```python
from build123d import *

# Parameters (mm, degrees)
F0_W      = 132.275518
F0_H      = 83.935342
F1_DEPTH  = 25.4
F1_FACE_W = 132.275518
F1_FACE_H = 83.935342
F2_DEPTH  = 39.878
F3_T      = -2.54


with BuildPart() as f1:
    # F0 (on Front) → F1 (new body)
    with BuildSketch(Plane.XZ):
        with Locations((5.538398, -30.956518)):
            Rectangle(F0_W, F0_H)
    extrude(amount=F1_DEPTH)

    # F1_face (on face) → F2 (join)
    with BuildSketch(Plane(origin=(5.538398, 0, -30.956518), x_dir=(1, 0, 0), z_dir=(0, 1, 0))):
        Rectangle(F1_FACE_W, F1_FACE_H)
    extrude(amount=F2_DEPTH)

    # F3
    f3_openings = [f1.faces().sort_by_distance(p)[0] for p in [
        (5.538398, 39.878, -30.956518),
    ]]
    offset(amount=F3_T, openings=f3_openings)


solid = f1.part
```
The model under review builds one solid part; all positions refer to its coordinate system, in mm. A direction names the side the tool comes from. Round coordinates to 2 decimals unless told otherwise and drop trailing zeros. Loops run counter-clockwise (first coordinate to the right, second up) from the corner with the lowest first, then second, coordinate; pieces in that order, holes last.
1) Clearance check with a flat-ended pin moving along its axis: P1, Ø3, axis at x = -1, z = -49, coming from the +Y side. State where the tip first meets the part, or that it passes through.
Values follow:
P1: stops at y = -22.86
2) Consider section A-A on y = 15.5. State the section outline as (x, z) points, then the cut area to 3 significant figures.
Values follow:
outline: (-60.6, -72.92) - (71.68, -72.92) - (71.68, 11.01) - (-60.6, 11.01) - close; hole (-58.06, -70.38) - (69.14, -70.38) - (69.14, 8.47) - (-58.06, 8.47) - close
area: 1,070 mm2
3) Wall thickness on line 1 along X through (y, z) = (-21, -36); line 2 along Z through (x, y) = (30.5, 5); line 3 along Y through (x, z) = (54, -48): over which ranges is each line inside the solid? List them lowest first.
Values follow:
line 1: x = -60.6 to -58.06, 69.14 to 71.68
line 2: z = -72.92 to -70.38, 8.47 to 11.01
line 3: y = -25.4 to -22.86
4) Tool access review of faces 1 (the face through (5, -22.86, -30)), 2 (the face through (-60.599, 7, -30)): name each direction out of +Z, -Z, +X, -X, +Y, -Y from which nothing blocks a thin tool from reaching the whole face with its end or side.
Values follow:
face 1: +Y
face 2: +Z, -Z, -X, +Y, -Y
5) The part is to be moulded in two halves that separate along Z. For faces 3 (the face through (5, 7, 11.011)), 4 (the face through (5, 7, -72.924)), 5 (the face through (69.136, 8, -30)), 6 (the face through (-14, 39.878, 9)), say which applies: pulls with the +Z half, pulls with the -Z half, needs draft (parallel to the pull), parting line crosses it, or undercut.
Values follow:
face 3: pulls with the +Z half
face 4: pulls with the -Z half
face 5: undercut
face 6: needs draft
6) Consider section B-B on z = -6. State the section outline as (x, y) points, then the cut area to 3 significant figures.
Values follow:
outline: (-60.6, -25.4) - (71.68, -25.4) - (71.68, 39.88) - (69.14, 39.88) - (69.14, -22.86) - (-58.06, -22.86) - (-58.06, 39.88) - (-60.6, 39.88) - close
area: 655 mm2
7) Consider section C-C on x = 1. State the section outline as (y, z) points, then the cut area to 3 significant figures.
Values follow:
outline: (-25.4, -72.92) - (39.88, -72.92) - (39.88, -70.38) - (-22.86, -70.38) - (-22.86, 8.47) - (39.88, 8.47) - (39.88, 11.01) - (-25.4, 11.01) - close
area: 532 mm2
